Here's the drawing with two shaded views (mm, measured from the low corner). I have some questions. A direction names the side the tool comes from. Round coordinates to 2 decimals unless told otherwise and drop trailing zeros. Write each loop counter-clockwise with the first axis right and the second up, starting at its lowest first coordinate (ties: lowest second). Pieces come first, ordered by that corner, then holes. Notation, with made-up numbers: M 20.5,88 L 28.5,88 A27 cw 28.5,112 Z; hole C 22.5,73 d1. An arc over 180 degrees is marked long. Answer as a JSON object with one key per item and string values. Group by question number.
1) Suppose I cut it at C-C, the plane y = 5.25. Write out the boundary of the cut face in (x, z).
2) Suppose I cut it at D-D, the plane y = 3.25. Write out the boundary of the cut face in (x, z), and give its area (3 significant figures).
3) On a 3-axis mill with a long thin cutter (end or side, diameter ignored), from which of +Z, -Z, +X, -X, +Y, -Y can I reach the whole of each face in a straight line? I mean the marked faces 4 and 5. Say none if no direction works.
4) I'm going to push flat-ended pins straight in: pin 1 Ø1 at (x, z) = (5, 5.5) entering from -Y; pin 2 Ø1.5 at (x, z) = (3.5, 1.5) entering from -Y; pin 3 Ø1.5 at (x, y) = (1.5, 7.5) entering from +Z; pin 4 Ø1.5 at (y, z) = (2.5, 2.5) entering from +X. Where does each tip first touch, or does it pass through?
5) Suppose I cut it at B-B, the plane z = 3.5. Write out the boundary of the cut face in (x, y) (3 decimals), and give its area (4 significant figures).
6) Suppose I cut it at A-A, the plane x = 3.5. Write out the boundary of the cut face in (y, z) (3 decimals).
7) Please list where these lines run through material, in increasing order: L1, parallel to X at y = 7.95, z = 3.5; L2, parallel to Y at x = 3.5, z = 4.25. Write a range as [from, to].
8) If we mould it in two halves opening along Z, with no side actions, what happens to the marked faces 1, 2 and 3? For each: +Z half, -Z half, draft (parallel to the pull), parting line (faces both ways), or undercut.
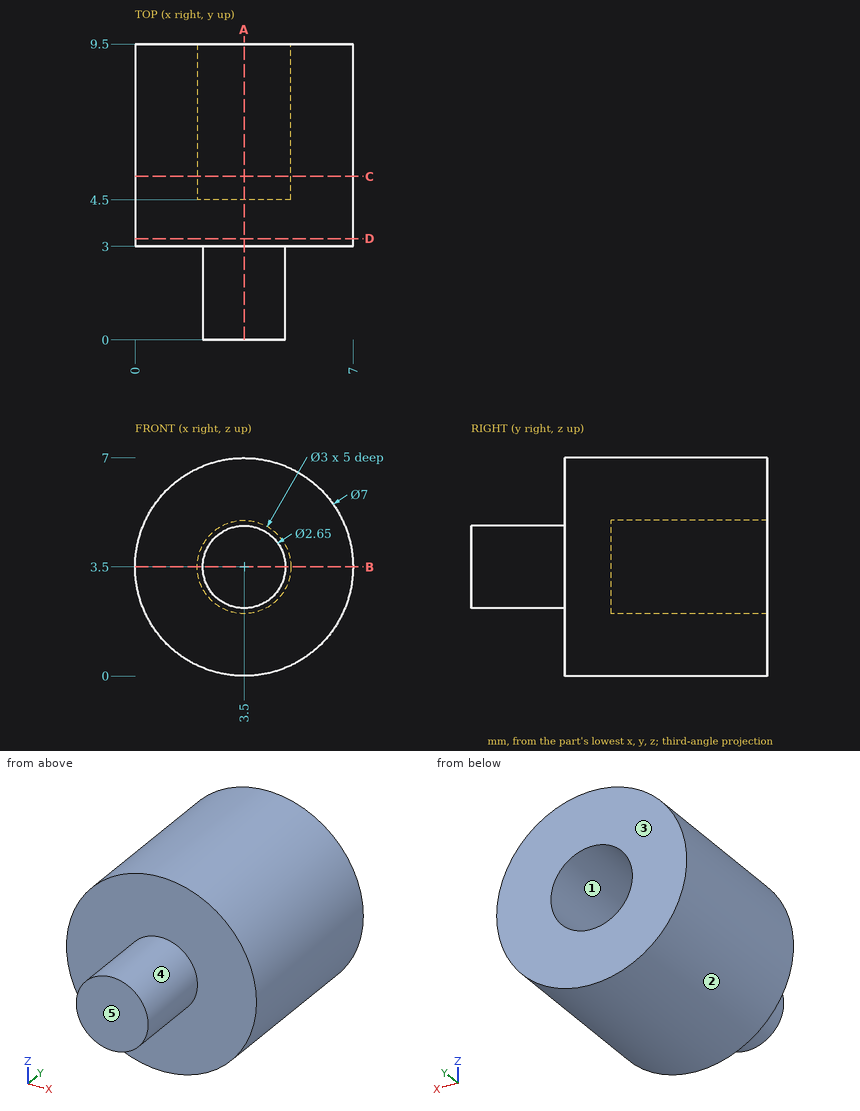
Results:
{
 "1": {"outline": "C 3.5,3.5 d7; hole C 3.5,3.5 d3"},
 "2": {"outline": "C 3.5,3.5 d7", "area": "38.5 mm^2"},
 "3": {"face 4": "-Y", "face 5": "+Z, -Z, +X, -X, -Y"},
 "4": {"pin 1": "y = 3", "pin 2": "y = 0", "pin 3": "z = 6.77", "pin 4": "x = 6.97"},
 "5": {"outline": "M 0,3 L 2.175,3 L 2.175,0 L 4.825,0 L 4.825,3 L 7,3 L 7,9.5 L 5,9.5 L 5,4.5 L 2,4.5 L 2,9.5 L 0,9.5 Z", "area": "38.45 mm^2"},
 "6": {"outline": "M 0,2.175 L 3,2.175 L 3,0 L 9.5,0 L 9.5,2 L 4.5,2 L 4.5,5 L 9.5,5 L 9.5,7 L 3,7 L 3,4.825 L 0,4.825 Z"},
 "7": {"L1": "[0, 2], [5, 7]", "L2": "[0, 4.5]"},
 "8": {"face 1": "undercut", "face 2": "parting line", "face 3": "draft"}
}
